Input: part model. Units: mm. Frame: model coordinates. Face numbers are marked on the shaded views. A direction names the side the tool comes from. Give positions to 0.01 mm unless a question says otherwise; leave off trailing zeros. Order: outer loops, then holes, each group sorted by start corner. A loop starts at its lowest first (then second) coordinate and runs counter-clockwise, first axis right, second up. Notation, with made-up numbers: (19.5, -34.5) - (57.5, -34.5) arc R3 ccw to (57.5, -30.5) - close; hole circle Ø8 at (67, -21.75). An arc over 180 degrees is marked (long way). Answer in a Markdown table with one row per item. Add a question column.
1. Ray query, line 1 (X direction, y = 31.5, z = 1.5); line 2 (Y direction, x = 9, z = 16.5); line 3 (Y direction, x = 31, z = 4.5). Return the intervals inside material, ascending. Write a range as [from, to].
2. Section query D-D on x = 55. Return loops of the section in (y, z), and give its area (3 significant figures).
3. Access query for the marked faces 1 and 2. Directions: +Z, -Z, +X, -X, +Y, -Y. A direction counts if a zero-diameter tool reaches every point of the face in a straight line with its end or side. Return the directions, or none.
4. Mould query, pull axis X, two halves, no side actions, for the marked faces 3, 4, 5 and 6. Classes: released by +X, released by -X, zero draft, split by the parting line, or undercut.
5. Contact query for flat-ended pins moving along their axis: pin 1 (1 mm diameter, centred on x = 39, y = 22.5, fed in from +Z); pin 2 (6.5 mm diameter, centred on y = 26, z = 24, fed in from +X). Output: stop coordinate, or through.
6. Section query C-C on y = 36.5. Return loops of the section in (x, z).
7. Section query B-B on y = 9. Return loops of the section in (x, z), and give its area (3 significant figures).
8. Section query A-A on z = 24. Return loops of the section in (x, y), and give its area (3 significant figures).
Autodesk Inventor part; units mm, degrees
ref_plane "YZ Plane" through (0, 0, 0) normal (1, 0, 0) x (0, 1, 0)
ref_plane "XZ Plane" through (0, 0, 0) normal (0, 1, 0) x (-1, 0, 0)
ref_plane "XY Plane" through (0, 0, 0) normal (0, 0, 1) x (1, 0, 0)
sketch "Sketch1" plane through (0, 0, 0) normal (0, 0, 1) x (1, 0, 0)
  line L0 (0, 0) -> (83.9978, 0)
  line L1 (83.9978, 0) -> (83.9978, 56.9999)
  line L2 (83.9978, 56.9999) -> (0, 56.9999)
  line L3 (0, 56.9999) -> (0, 0)
  dimension "d0" = 83.9978
  dimension "d1" = 56.9999
extrude "Extrusion1" add sketch "Sketch1" along normal blind 29.9999
shell "Shell1" thickness 2 outward yes removed faces 1 at (27.9993, 37.9999, 29.9999)
sketch "Sketch2" plane through (85.9978, -2, -2) normal (1, 0, 0) x (0, 0, -1)
  point P0 (-2, 2)
sketch "Sketch3" plane through (85.9978, -2, -2) normal (1, 0, 0) x (0, 0, -1)
  line L0 (-2, 58.9999) -> (-31.9999, 58.9999)
  line L1 (-29.6685, 58.1425) -> (-23.6741, 58.1425)
  line L2 (-23.6741, 58.1425) -> (-23.6741, 2.1426)
  line L3 (-23.6741, 2.1426) -> (-29.6685, 2.1426)
  line L4 (-29.6685, 2.1426) -> (-29.6685, 58.1425)
  point P0 (-2, 2)
  dimension "d5" = 5.9944
  dimension "d6" = 55.9999
extrude "Extrusion2" cut sketch "Sketch3" against normal blind 87.0001
sketch "Sketch4" plane through (85.9978, -2, -2) normal (1, 0, 0) x (0, 0, -1)
  line L0 (-14.3813, 35.0012) -> (-18.3691, 35.0012)
  line L1 (-18.3691, 35.0012) -> (-18.3691, 43.5102)
  line L2 (-18.3691, 43.5102) -> (-14.3813, 43.5102)
  line L3 (-14.3813, 43.5102) -> (-14.3813, 35.0012)
  point P0 (-2, 2)
  point P1 (-13.7922, 50.8)
  dimension "d9" = 3.9878
  dimension "d10" = 8.509
extrude "Extrusion3" cut sketch "Sketch4" against normal blind 12.7
sketch "Sketch5" plane through (-2, 58.9999, -2) normal (0, 1, 0) x (1, 0, 0)
  line L0 (85.9978, -31.9999) -> (2, -31.9999)
  line L1 (31.9983, -31.9999) -> (35.9099, -31.9999)
  line L2 (35.9099, -31.9999) -> (35.9099, -2)
  line L3 (35.9099, -2) -> (31.9983, -2)
  line L4 (31.9983, -2) -> (31.9983, -31.9999)
  point P0 (2, -2)
  dimension "d13" = 3.9116
extrude "Extrusion4" cut sketch "Sketch5" against normal blind 12.7
properties part number "case-v3"
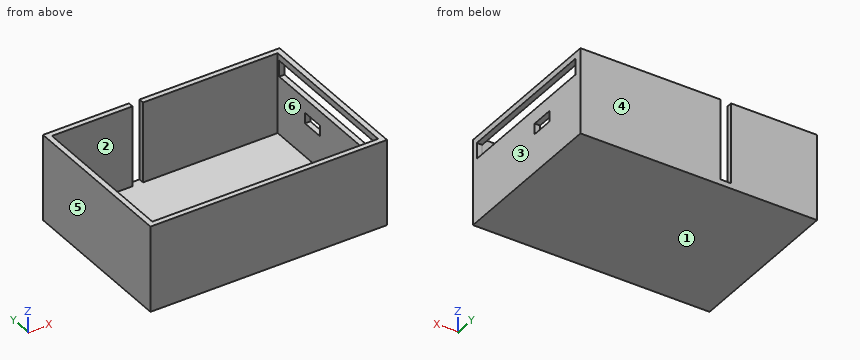
Answer:
| question | item | result |
|---|---|---|
| 1 | line 1 | x = [-2, 0], [84, 86] |
| 1 | line 2 | y = [-2, 0], [57, 59] |
| 1 | line 3 | y = [-2, 0] |
| 2 | outline | (-2, -2) - (59, -2) - (59, 30) - (57, 30) - (57, 0) - (0, 0) - (0, 30) - (-2, 30) - close |
| 2 | area | 242 mm² |
| 3 | face 1 | -Z, +X, -X, +Y, -Y |
| 3 | face 2 | +Z |
| 4 | face 3 | released by +X |
| 4 | face 4 | zero draft |
| 4 | face 5 | released by -X |
| 4 | face 6 | undercut |
| 5 | pin 1 | stops at z = 0 |
| 5 | pin 2 | stops at x = 86 |
| 6 | outline | (-2, -2) - (86, -2) - (86, 12.38) - (84, 12.38) - (84, 0) - (0, 0) - (0, 21.67) - (-1, 21.67) - (-1, 27.67) - (0, 27.67) - (0, 30) - (-2, 30) - close; (84, 16.37) - (86, 16.37) - (86, 21.67) - (84, 21.67) - close; (84, 27.67) - (86, 27.67) - (86, 30) - (84, 30) - close |
| 7 | outline | (-2, -2) - (86, -2) - (86, 21.67) - (84, 21.67) - (84, 0) - (0, 0) - (0, 21.67) - (-1, 21.67) - (-1, 27.67) - (0, 27.67) - (0, 30) - (-2, 30) - close; (84, 27.67) - (86, 27.67) - (86, 30) - (84, 30) - close |
| 7 | area | 278 mm² |
| 8 | outline | (-2, -2) - (86, -2) - (86, 0.14) - (84, 0.14) - (84, 0) - (0, 0) - (0, 0.14) - (-1, 0.14) - (-1, 56.14) - (0, 56.14) - (0, 57) - (30, 57) - (30, 59) - (-2, 59) - close; (33.91, 57) - (84, 57) - (84, 56.14) - (86, 56.14) - (86, 59) - (33.91, 59) - close |
| 8 | area | 404 mm² |
